Input: part model. Units: mm. Frame: model coordinates. A direction names the side the tool comes from. Give positions to 0.01 mm unless a question says otherwise; leave off trailing zeros. Loops run counter-clockwise (first coordinate to the right, second up) from the corner with the lowest first, then second, coordinate; pieces in that order, holes last. Notation, with made-up numbers: M 32,37.25 L 48,37.25 A21 cw 48,64.25 Z; hole C -29.5,5 d9. An arc over 180 degrees is marked long. Use a Markdown table: item, result. Add a question column.
from build123d import *

# Parameters (mm, degrees)
SKETCH1_R           = 3.175
BOSS_EXTRUDE1_DEPTH = 12.7
SKETCH2_W           = 8.128
SKETCH2_H           = 3.048
BOSS_EXTRUDE2_DEPTH = 8.255


with BuildPart() as part:
    # Sketch1 → Boss-Extrude1 (new body, symmetric)
    with BuildSketch(Plane(origin=(0, 0, 0), x_dir=(1, 0, 0), z_dir=(0, 1, 0))):
        Circle(SKETCH1_R)
    extrude(amount=BOSS_EXTRUDE1_DEPTH, both=True)

    # Sketch2 → Boss-Extrude2 (add, symmetric)
    with BuildSketch(Plane(origin=(0, 0, 0), x_dir=(1, 0, 0), z_dir=(0, 1, 0))):
        Rectangle(SKETCH2_W, SKETCH2_H)
    extrude(amount=BOSS_EXTRUDE2_DEPTH, both=True)


solid = part.part
1) Section query B-B, the plane y = -7. Return the cut outline in (x, z) (3 decimals), and give its area (3 significant figures).
2) Section query C-C, the plane x = -0.75. Return the cut outline in (y, z).
3) Section query A-A, the plane z = 0. Return the cut outline in (x, y) (3 decimals).
4) Section query D-D, the plane z = 2.25. Return the cut outline in (x, y).
5) Ray query, line 1 (Z direction, x = -3, y = -4.75); line 2 (Y direction, x = -3.25, z = 0.25) (3 decimals); line 3 (Z direction, x = 2.75, y = 9.75). Return the intervals inside material, ascending. Write a range as [from, to].
6) Contact query for flat-ended pins moving along their axis: P1, Ø0.6, axis at x = -3.5, z = -0.5, coming from the -Y side (3 decimals); P2, Ø2, axis at x = -3, y = -3.5, coming from the -Z side; P3, Ø0.6, axis at x = 3.5, z = -0.5, coming from the +Y side (3 decimals). Output: stop coordinate, or through.
7) Reachability of faces 1 (the flat face through (-3, 0, -1.524)), 2 (the flat face through (-3, 0, 1.524)), 3 (the flat face through (3, 0, -1.524)), 4 (the flat face through (-4.064, 0, 0)), 5 (the flat face through (3, 0, 1.524)) from +Z, -Z, +X, -X, +Y, -Y: full face, straight path, thin tool, end or side. Return the list, or none.
Entries:
| question | item | result |
|---|---|---|
| 1 | outline | M -4.064,-1.524 L -2.785,-1.524 A3.175 ccw 2.785,-1.524 L 4.064,-1.524 L 4.064,1.524 L 2.785,1.524 A3.175 ccw -2.785,1.524 L -4.064,1.524 Z |
| 1 | area | 37.9 mm² |
| 2 | outline | M -12.7,-3.09 L 12.7,-3.09 L 12.7,3.09 L -12.7,3.09 Z |
| 3 | outline | M -4.064,-8.255 L -3.175,-8.255 L -3.175,-12.7 L 3.175,-12.7 L 3.175,-8.255 L 4.064,-8.255 L 4.064,8.255 L 3.175,8.255 L 3.175,12.7 L -3.175,12.7 L -3.175,8.255 L -4.064,8.255 Z |
| 4 | outline | M -2.24,-12.7 L 2.24,-12.7 L 2.24,12.7 L -2.24,12.7 Z |
| 5 | line 1 | z = [-1.52, 1.52] |
| 5 | line 2 | y = [-8.255, 8.255] |
| 5 | line 3 | z = [-1.59, 1.59] |
| 6 | P1 | stops at y = -8.255 |
| 6 | P2 | stops at z = -2.47 |
| 6 | P3 | stops at y = 8.255 |
| 7 | face 1 | -Z, -X, +Y, -Y |
| 7 | face 2 | +Z, -X, +Y, -Y |
| 7 | face 3 | -Z, +X, +Y, -Y |
| 7 | face 4 | +Z, -Z, -X, +Y, -Y |
| 7 | face 5 | +Z, +X, +Y, -Y |
